Source: three-view drawing plus pictorial views. Frame: mm from the lowest corner of the part. Give positions to 0.01 mm unless a question says otherwise; leave off trailing zeros. Loops run counter-clockwise (first coordinate to the right, second up) from the corner with the lowest first, then second, coordinate; pieces in that order, holes last. Notation, with made-up numbers: M 47,30 L 76,30 A8 cw 76,42 Z; hole C 30.25,85 d1. An arc over 180 degrees is marked long. One line per item, written item: value. Start each with the question number.
(1) Section A-A on x = 5. Output: boundary loops of the cut face in (y, z).
(2) Ray query, line 1 along Z through (x, y) = (5, 1.35); line 2 along X through (y, z) = (1.15, 5); line 3 along X through (y, z) = (1.35, 6). Return the intervals inside material, ascending. Write a range as from..to.
(3) Section B-B on y = 0.65. Output: boundary loops of the cut face in (x, z), plus the area to 3 significant figures.
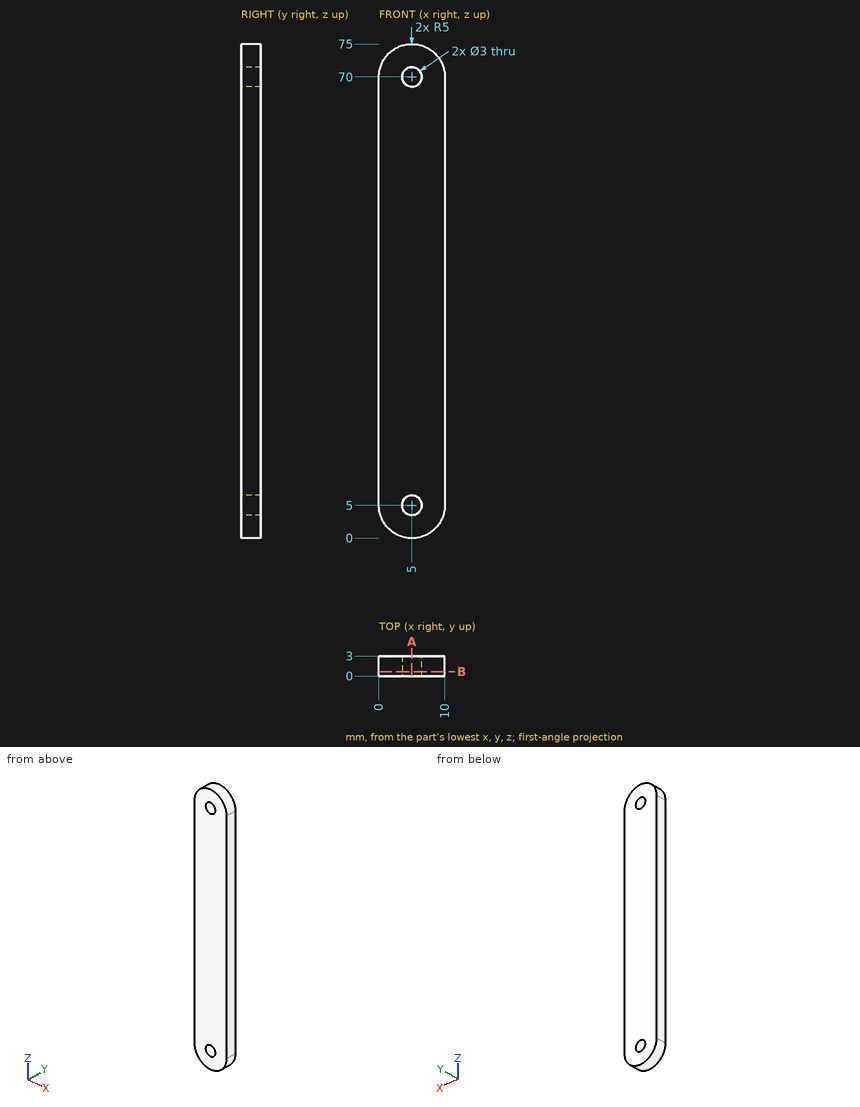
Output values:
1. outline: M 0,0 L 3,0 L 3,3.5 L 0,3.5 Z; M 0,6.5 L 3,6.5 L 3,68.5 L 0,68.5 Z; M 0,71.5 L 3,71.5 L 3,75 L 0,75 Z
2. line 1: z = 0..3.5, 6.5..68.5, 71.5..75
2. line 2: x = 0..3.5, 6.5..10
2. line 3: x = 0..3.88, 6.12..10
3. outline: M 0,5 A5 ccw 10,5 L 10,70 A5 ccw 0,70 Z; hole C 5,5 d3; hole C 5,70 d3
3. area: 714 mm²
